Input: part model. Units: mm. Frame: model coordinates. A direction names the side the tool comes from. Round coordinates to 2 decimals unless told otherwise and drop trailing zeros. Write each loop counter-clockwise with the first axis right and the second up, starting at its lowest first coordinate (ties: lowest second). Pieces come first, ordered by that corner, then holes. Notation, with made-up numbers: (85, 6.5) - (104, 6.5) arc R17 cw to (104, 38.5) - close; hole circle Ø11 at (-26, 8). An arc over 180 degrees is marked (long way). Use one line per item in the form item = value.
```python
from build123d import *

# Parameters (mm, degrees)
SKETCH015_W     = 31
SKETCH015_H     = 150
PAD010_DEPTH    = 13
SKETCH016_W     = 12
SKETCH016_H     = 10
POCKET004_DEPTH = 5
SKETCH017_R     = 4
PAD011_DEPTH    = 10


with BuildPart() as part:
    # Sketch015 → Pad010 (new body)
    with BuildSketch(Plane.XY):
        with Locations((15.5, 75)):
            Rectangle(SKETCH015_W, SKETCH015_H)
    extrude(amount=PAD010_DEPTH)

    # Sketch016 (on Face1 of Pad010) → Pocket004 (cut)
    with BuildSketch(Plane.XZ):
        with Locations((16, 6)):
            Rectangle(SKETCH016_W, SKETCH016_H)
    extrude(amount=-POCKET004_DEPTH, mode=Mode.SUBTRACT)

    # Sketch017 (on Face10 of Pocket004) → Pad011 (join)
    with BuildSketch(Plane(origin=(0, 150, 0), x_dir=(-1, 0, 0), z_dir=(0, 1, 0))):
        with Locations((-15, 6)):
            Circle(SKETCH017_R)
    extrude(amount=PAD011_DEPTH)


with BuildPart() as part_1:
    # Body008 placement: moved
    add(part.part.moved(Location((25, 37, -13.2))))


solid = part_1.part
```
(1) Cut plane B-B on x = 40. Output: boundary loops of the cut face in (y, z), then the cut area to 3 significant figures.
Derived:
outline = (37, -13.2) - (187, -13.2) - (187, -11.2) - (197, -11.2) - (197, -3.2) - (187, -3.2) - (187, -0.2) - (37, -0.2) - (37, -2.2) - (42, -2.2) - (42, -12.2) - (37, -12.2) - close
area = 1,980 mm^2
(2) Draft query along Z for faces 3 (the face through (56, 111, -7)), 4 (the face through (43.2, 191.9, -9.6)), 5 (the face through (35, 39, -7)). Return one class per face: released by +Z, released by -Z, zero draft, split by the parting line, or undercut.
Derived:
face_3 = zero draft
face_4 = split by the parting line
face_5 = undercut
(3) Cut plane C-C on x = 51. Output: boundary loops of the cut face in (y, z).
Derived:
outline = (37, -13.2) - (187, -13.2) - (187, -0.2) - (37, -0.2) - close
(4) Cut plane A-A on z = -7.2. Output: boundary loops of the cut face in (x, y), then the cut area to 3 significant figures.
Derived:
outline = (25, 37) - (35, 37) - (35, 42) - (47, 42) - (47, 37) - (56, 37) - (56, 187) - (44, 187) - (44, 197) - (36, 197) - (36, 187) - (25, 187) - close
area = 4,670 mm^2
(5) Material intervals for L1, parallel to Y at x = 50, z = -10; L2, parallel to Y at x = 45, z = -4.5; L3, parallel to X at y = 190, z = -5.5, sorted ascending.
Derived:
L1 = 37 to 187
L2 = 42 to 187
L3 = 36.38 to 43.62
(6) Access query for faces 1 (the face through (41, 39, -12.2)), 2 (the face through (40, 113, -13.2)). Directions: +Z, -Z, +X, -X, +Y, -Y. A direction counts if a zero-diameter tool reaches every point of the face in a straight line with its end or side. Return the directions, or none.
Derived:
face_1 = -Y
face_2 = -Z, +X, -X, +Y, -Y
